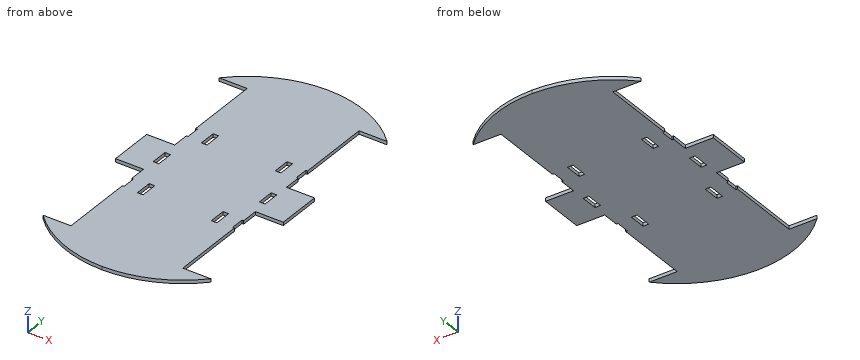
Autodesk Fusion 360 part; units mm, degrees
sketch "Sketch1" plane through (0, 0, 0) normal (0, 0, 1) x (1, 0, 0)
  line L0 (0, 0) -> (75, 0) construction
  line L1 (0, 0) -> (0, 145) construction
  line L2 (75, 0) -> (75, 20)
  line L3 (75, 20) -> (50, 20)
  line L4 (50, 20) -> (50, 113)
  line L5 (50, 113) -> (75, 113)
  arc A0 (75, 113) -> (0, 145) centre (0, 41.1094) ccw
  line L6 (0, 145) -> (-55.6559, 145) construction
  line L7 (-75, 0) -> (-75, 20)
  line L8 (-75, 20) -> (-50, 20)
  line L9 (-50, 20) -> (-50, 113)
  line L10 (-50, 113) -> (-75, 113)
  arc A1 (0, 145) -> (-75, 113) centre (0, 41.1094) ccw
  line L11 (75, 0) -> (75, -20)
  line L12 (75, -20) -> (50, -20)
  line L13 (50, -20) -> (50, -113)
  line L14 (50, -113) -> (75, -113)
  arc A2 (0, -145) -> (75, -113) centre (0, -41.1094) ccw
  line L15 (-50, -113) -> (-75, -113)
  line L16 (-50, -20) -> (-50, -113)
  line L17 (-75, -20) -> (-50, -20)
  line L18 (-75, 0) -> (-75, -20)
  arc A3 (-75, -113) -> (0, -145) centre (0, -41.1094) ccw
  line L19 (50, 35) -> (48.5, 35)
  line L20 (48.5, 35) -> (48.5, 47)
  line L21 (48.5, 47) -> (50, 47)
  line L22 (50, 47) -> (50, 35)
  line L23 (-50, 47) -> (-50, 35)
  line L24 (-50, 35) -> (-48.5, 35)
  line L25 (-48.5, 35) -> (-48.5, 47)
  line L26 (-48.5, 47) -> (-50, 47)
  line L27 (-48.5, -47) -> (-50, -47)
  line L28 (-50, -47) -> (-50, -35)
  line L29 (50, -47) -> (50, -35)
  line L30 (50, -35) -> (48.5, -35)
  line L31 (-50, -35) -> (-48.5, -35)
  line L32 (48.5, -35) -> (48.5, -47)
  line L33 (-48.5, -35) -> (-48.5, -47)
  line L34 (48.5, -47) -> (50, -47)
  line L35 (-50, 7.5) -> (-45, 7.5)
  line L36 (-45, 7.5) -> (-45, -7.5)
  line L37 (-45, -7.5) -> (-50, -7.5)
  line L38 (-50, -7.5) -> (-50, 7.5)
  line L39 (-45, 0) -> (0, 0) construction
  line L40 (50, 7.5) -> (45, 7.5)
  line L41 (45, 7.5) -> (45, -7.5)
  line L42 (45, -7.5) -> (50, -7.5)
  line L43 (50, -7.5) -> (50, 7.5)
  line L44 (-35.5, 48.5) -> (-30.5, 48.5)
  line L45 (-30.5, 48.5) -> (-30.5, 33.5)
  line L46 (-30.5, 33.5) -> (-35.5, 33.5)
  line L47 (-35.5, 33.5) -> (-35.5, 48.5)
  line L48 (-48.5, 41) -> (-35.5, 41) construction
  line L49 (30.5, 48.5) -> (30.5, 33.5)
  line L50 (30.5, 33.5) -> (35.5, 33.5)
  line L51 (35.5, 33.5) -> (35.5, 48.5)
  line L52 (35.5, 48.5) -> (30.5, 48.5)
  line L53 (-30.5, -48.5) -> (-30.5, -33.5)
  line L54 (-30.5, -33.5) -> (-35.5, -33.5)
  line L55 (-35.5, -33.5) -> (-35.5, -48.5)
  line L56 (-35.5, -48.5) -> (-30.5, -48.5)
  line L57 (35.5, -33.5) -> (35.5, -48.5)
  line L58 (35.5, -48.5) -> (30.5, -48.5)
  line L59 (30.5, -48.5) -> (30.5, -33.5)
  line L60 (30.5, -33.5) -> (35.5, -33.5)
  point P0 (35.5, 41)
  dimension "d6" = 75
  dimension "d7" = 145
  dimension "d8" = 20
  dimension "d9" = 25
  dimension "d10" = 93
  dimension "d11" = 15
  dimension "d12" = 1.5
  dimension "d13" = 12
  dimension "d15" = 5
  dimension "d16" = 15
  dimension "d17" = 25
  dimension "d18" = 5
  dimension "d19" = 15
  dimension "d20" = 13
extrude "Extrude1" add sketch "Sketch1" along normal blind 3 contours L2 L3 L4 L5 A0 L7 L8 L9 L10 A1 L11 L12 L13 L14 A2 L15 L16 L17 L18 A3 L19 L20 L21 L24 L25 L26 L27 L30 L31 L32 L33 L34
sketch "Sketch2" plane through (0, 0, 3) normal (0, 0, 1) x (-1, 0, 0)
  line L0 (-30.5, 48.5) -> (-30.5, 33.5)
  line L1 (-30.5, 33.5) -> (-35.5, 33.5)
  line L2 (-35.5, 33.5) -> (-35.5, 48.5)
  line L3 (-35.5, 48.5) -> (-30.5, 48.5)
  line L4 (45, 7.5) -> (50, 7.5)
  line L5 (50, 7.5) -> (50, -7.5)
  line L6 (50, -7.5) -> (45, -7.5)
  line L7 (45, -7.5) -> (45, 7.5)
  line L8 (30.5, 48.5) -> (35.5, 48.5)
  line L9 (35.5, 48.5) -> (35.5, 33.5)
  line L10 (35.5, 33.5) -> (30.5, 33.5)
  line L11 (30.5, 33.5) -> (30.5, 48.5)
  line L12 (-30.5, -48.5) -> (-35.5, -48.5)
  line L13 (-35.5, -48.5) -> (-35.5, -33.5)
  line L14 (-35.5, -33.5) -> (-30.5, -33.5)
  line L15 (-30.5, -33.5) -> (-30.5, -48.5)
  line L16 (30.5, -33.5) -> (35.5, -33.5)
  line L17 (35.5, -33.5) -> (35.5, -48.5)
  line L18 (35.5, -48.5) -> (30.5, -48.5)
  line L19 (30.5, -48.5) -> (30.5, -33.5)
  line L20 (-50, -7.5) -> (-50, 7.5)
  line L21 (-50, 7.5) -> (-45, 7.5)
  line L22 (-45, 7.5) -> (-45, -7.5)
  line L23 (-45, -7.5) -> (-50, -7.5)
  line L24 (-75, 20) -> (-75, -20)
  line L25 (-75, -20) -> (-50, -20)
  line L26 (-50, -20) -> (-50, -35)
  line L27 (-50, -35) -> (-48.5, -35)
  line L28 (-48.5, -35) -> (-48.5, -47)
  line L29 (-48.5, -47) -> (-50, -47)
  line L30 (-50, -47) -> (-50, -113)
  line L31 (-50, -113) -> (-75, -113)
  arc A0 (-75, -113) -> (75, -113) centre (0, -41.1094) ccw
  line L32 (75, -113) -> (50, -113)
  line L33 (50, -113) -> (50, -47)
  line L34 (50, -47) -> (48.5, -47)
  line L35 (48.5, -47) -> (48.5, -35)
  line L36 (48.5, -35) -> (50, -35)
  line L37 (50, -35) -> (50, -20)
  line L38 (50, -20) -> (75, -20)
  line L39 (75, -20) -> (75, 20)
  line L40 (75, 20) -> (50, 20)
  line L41 (50, 20) -> (50, 35)
  line L42 (50, 35) -> (48.5, 35)
  line L43 (48.5, 35) -> (48.5, 47)
  line L44 (48.5, 47) -> (50, 47)
  line L45 (50, 47) -> (50, 113)
  line L46 (50, 113) -> (75, 113)
  arc A1 (75, 113) -> (-75, 113) centre (0, 41.1094) ccw
  line L47 (-75, 113) -> (-50, 113)
  line L48 (-50, 113) -> (-50, 47)
  line L49 (-50, 47) -> (-48.5, 47)
  line L50 (-48.5, 47) -> (-48.5, 35)
  line L51 (-48.5, 35) -> (-50, 35)
  line L52 (-50, 35) -> (-50, 20)
  line L53 (-50, 20) -> (-75, 20)
equation "d6 = ( 150 / 2 ) * 1 mm"
equation "d7 = ( 290 / 2 ) * 1 mm"
equation "d8 = ( 40 / 2 ) * 1 mm"
Design review of the part built by this model. Coordinates are the model's own, in mm. Coordinates: 2 decimals unless noted, no trailing zeros. Loops run counter-clockwise (first coordinate to the right, second up) from the corner with the lowest first, then second, coordinate; pieces in that order, holes last.
Q1. We need section D-D on y = -92.5. State the section outline as (x, z) points, and give its area (3 significant figures).
Reported:
outline: (-50, 0) - (50, 0) - (50, 3) - (-50, 3) - close
area: 300 mm2
Q2. To check wall thickness, follow line 1 (X direction, y = -45.5, z = 1.4); line 2 (Y direction, x = -57, z = 0.7); line 3 (Y direction, x = -58.5, z = 1.95). State the ranges of each line that lie inside material, in increasing order.
Reported:
line 1: x = -48.5 to -35.5, -30.5 to 30.5, 35.5 to 48.5
line 2: y = -127.97 to -113, -20 to 20, 113 to 127.97
line 3: y = -126.96 to -113, -20 to 20, 113 to 126.96
Q3. For pin 1 (1.5 mm diameter, centred on x = 32, z = 1, fed in from -Y); pin 2 (1.5 mm diameter, centred on x = 66.5, z = 1.5, fed in from -Y); pin 3 (1.5 mm diameter, centred on y = -86.5, z = 0.5, fed in from -X), all flat-tipped, find the tip position at first contact; note any pin that passes through.
Reported:
pin 1: stops at y = -140.19
pin 2: stops at y = -121.55
pin 3: stops at x = -50
Q4. We need section A-A on y = 41. State the section outline as (x, z) points, and give its area (3 significant figures).
Reported:
outline: (-48.5, 0) - (-35.5, 0) - (-35.5, 3) - (-48.5, 3) - close; (-30.5, 0) - (30.5, 0) - (30.5, 3) - (-30.5, 3) - close; (35.5, 0) - (48.5, 0) - (48.5, 3) - (35.5, 3) - close
area: 261 mm2
Q5. We need section B-B on x = 61. State the section outline as (y, z) points.
Reported:
outline: (-125.21, 0) - (-113, 0) - (-113, 3) - (-125.21, 3) - close; (-20, 0) - (20, 0) - (20, 3) - (-20, 3) - close; (113, 0) - (125.21, 0) - (125.21, 3) - (113, 3) - close
Q6. We need section C-C on z = 1.4. State how many separate pieces and enclosed holes the cut face has, and give its area (3 significant figures).
Reported:
separate pieces: 1
enclosed holes: 6
area: 30,700 mm2
